Read the model definition and answer for the solid it produces. Units are mm, in the model's axes. Give positions to 0.01 mm unless a question says otherwise; leave off trailing zeros. Loops run counter-clockwise (first coordinate to the right, second up) from the corner with the lowest first, then second, coordinate; pieces in that order, holes last.
(1) Find section A-A, the plane z = 6.35. Write down the section's boundary in (x, y) (1 decimal), then the cut area to 3 significant figures.
(2) Find section C-C, the plane y = 2.45. State how many separate pieces and enclosed holes the cut face has, then the cut area to 3 significant figures.
(3) Find section B-B, the plane x = -25.4. Write down the section's boundary in (y, z) (3 decimals).
(4) Straight lines are drawn through the part: probe 1 along X at (y, z) = (1.4, 2.5); probe 2 along X at (y, z) = (1.2, -0.5); probe 3 along X at (y, z) = (2.4, 6.35). For each, find the intervals that lie inside material, in ascending order.
(5) Find section D-D, the plane z = 0. Write down the section's boundary in (x, y) (3 decimals), then the cut area to 3 significant figures.
```python
from build123d import *

# Parameters (mm, degrees)
SKETCH2_W           = 101.6
SKETCH2_H           = 43.18
SKETCH2_R           = 1.4605
SKETCH2_R_2         = 3.175
BOSS_EXTRUDE1_DEPTH = 3.175


with BuildPart() as part:
    # Sketch2 → Boss-Extrude1 (new body)
    with BuildSketch(Plane(origin=(0, 0, 0), x_dir=(1, 0, 0), z_dir=(0, 1, 0))):
        with Locations((0, -3.81)):
            Rectangle(SKETCH2_W, SKETCH2_H)
        with Locations(Location((0, -6.35, 0), (0, 0, 270))):
            Circle(SKETCH2_R, mode=Mode.SUBTRACT)
        with Locations(Location((-25.4, 0, 0), (0, 0, 270))):
            Circle(SKETCH2_R_2, mode=Mode.SUBTRACT)
        with BuildLine():
            ThreePointArc((22.225, 0), (25.4, 3.175), (28.575, 0))
            ThreePointArc((28.575, 0), (25.4, -3.175), (22.225, 0))
        make_face(mode=Mode.SUBTRACT)
    extrude(amount=BOSS_EXTRUDE1_DEPTH)


solid = part.part
```
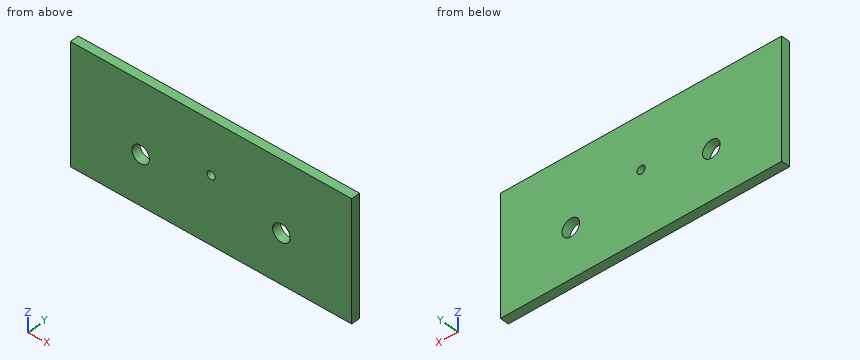
Entries:
1. outline: (-50.8, 0) - (-1.5, 0) - (-1.5, 3.2) - (-50.8, 3.2) - close; (1.5, 0) - (50.8, 0) - (50.8, 3.2) - (1.5, 3.2) - close
1. area: 313 mm2
2. separate pieces: 1
2. enclosed holes: 3
2. area: 4,320 mm2
3. outline: (0, -17.78) - (3.175, -17.78) - (3.175, -3.175) - (0, -3.175) - close; (0, 3.175) - (3.175, 3.175) - (3.175, 25.4) - (0, 25.4) - close
4. probe 1: x = -50.8 to -27.36, -23.44 to 23.44, 27.36 to 50.8
4. probe 2: x = -50.8 to -28.54, -22.26 to 22.26, 28.54 to 50.8
4. probe 3: x = -50.8 to -1.46, 1.46 to 50.8
5. outline: (-50.8, 0) - (-28.575, 0) - (-28.575, 3.175) - (-50.8, 3.175) - close; (-22.225, 0) - (22.225, 0) - (22.225, 3.175) - (-22.225, 3.175) - close; (28.575, 0) - (50.8, 0) - (50.8, 3.175) - (28.575, 3.175) - close
5. area: 282 mm2
